Here's the drawing with two shaded views (mm, measured from the low corner). I have some questions. Round coordinates to 2 decimals unless told otherwise and drop trailing zeros. Loops run counter-clockwise (first coordinate to the right, second up) from the corner with the lowest first, then second, coordinate; pieces in that order, holes last. Notation, with made-up numbers: (65, -5.75) -> (102, -5.75) arc R19 cw to (102, 8.25) -> close; hole circle Ø1 at (-24, 86). An arc over 180 degrees is marked (long way). Write each question's results on one line, items separated by ' | '. Start each with the question number.
1) Imagine slicing it at A-A, the plane z = 41. List the corners of the cut face in (x, y) for me, plus the area to 3 significant figures.
2) Imagine slicing it at B-B, the plane x = 99. List the corners of the cut face in (y, z) for me, plus the area to 3 significant figures.
3) For P1, Ø2, axis at x = 33, y = 1, coming from the -Z side; P2, Ø3, axis at x = 58, z = 57, coming from the +Y side, each with a flat end and sliding along its axis, tell me the tip position at first contact or that it passes through.
4) If I drill on probe 1 along X at (y, z) = (1.4, 112.5); probe 2 along Z at (x, y) = (3.5, 2.2); probe 3 along Z at (x, y) = (150.5, 1.1), over which ranges is the centre line in solid material (lowest first)?
5) We'd pull the mould along Z, two halves only. Please class the marked faces 1 and 2: pulls with the +Z half, pulls with the -Z half, needs draft (parallel to the pull), parting line crosses it, or undercut.
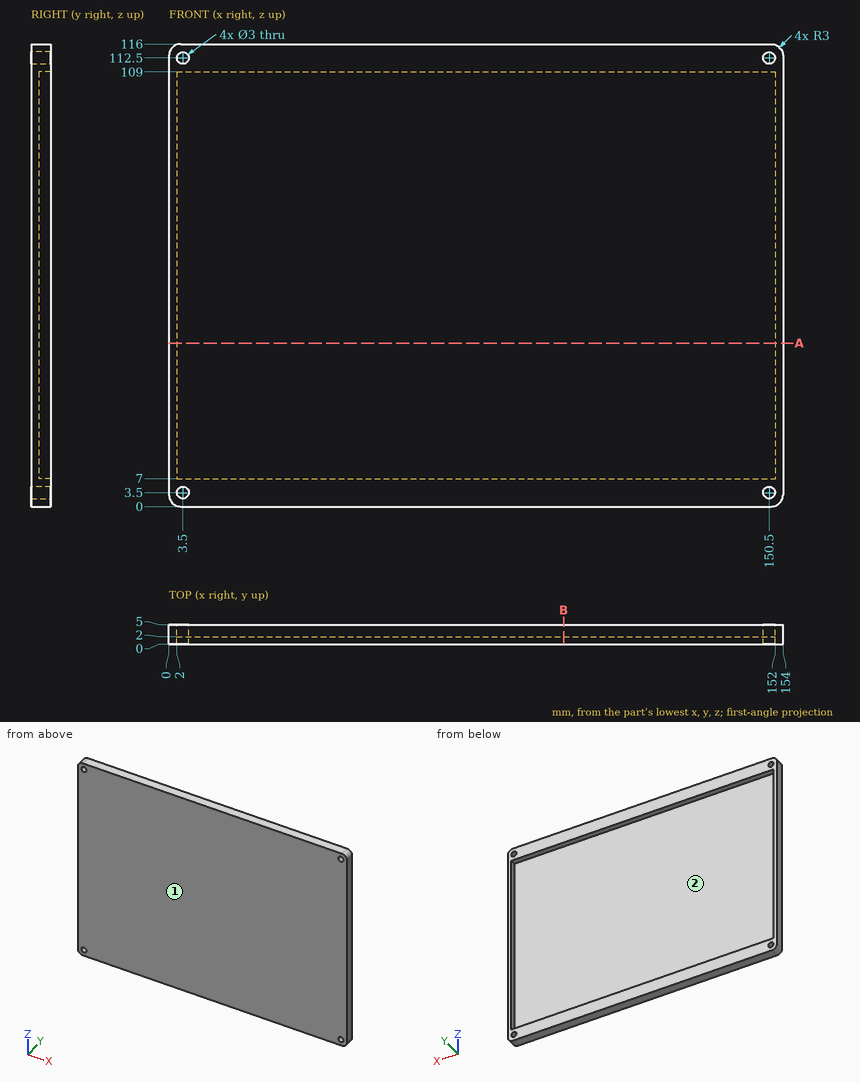
Checked values:
1) outline: (0, 0) -> (154, 0) -> (154, 5) -> (152, 5) -> (152, 2) -> (2, 2) -> (2, 5) -> (0, 5) -> close | area: 320 mm^2
2) outline: (0, 0) -> (5, 0) -> (5, 7) -> (2, 7) -> (2, 109) -> (5, 109) -> (5, 116) -> (0, 116) -> close | area: 274 mm^2
3) P1: z = 0 | P2: y = 2
4) probe 1: 0 to 2, 5 to 149, 152 to 154 | probe 2: 0 to 2, 5 to 7, 109 to 111, 114 to 116 | probe 3: 0 to 2, 5 to 111, 114 to 116
5) face 1: needs draft | face 2: undercut
